from build123d import *

# Parameters (mm, degrees)
BOSS_EXTRUDE1_DEPTH = 3
SKETCH2_R           = 1.5
CUT_EXTRUDE3_DEPTH  = 3
CUT_EXTRUDE4_START  = -10
CUT_EXTRUDE4_DEPTH  = 10
BOSS_EXTRUDE2_START = -3
BOSS_EXTRUDE2_DEPTH = 3
SKETCH5_W           = 0.56
SKETCH5_H           = 32.898596714
CUT_EXTRUDE5_DEPTH  = 3
SKETCH6_W           = 0.2
SKETCH6_H           = 32.898596714
CUT_EXTRUDE6_DEPTH  = 3
SKETCH7_R           = 2
CUT_EXTRUDE8_DEPTH  = 3
BOSS_EXTRUDE3_START = -3
BOSS_EXTRUDE3_DEPTH = 3
CUT_EXTRUDE9_START  = -3
CUT_EXTRUDE9_DEPTH  = 3
BOSS_EXTRUDE5_START = -3
BOSS_EXTRUDE5_DEPTH = 3
SKETCH11_R          = 1.5
CUT_EXTRUDE10_DEPTH = 3
CUT_EXTRUDE11_DEPTH = 3
SKETCH13_W          = 7
SKETCH13_H          = 1.5
CUT_EXTRUDE12_DEPTH = 3
SKETCH14_R          = 2
SKETCH14_R_2        = 1.5
SKETCH14_W          = 7
SKETCH14_H          = 1.5
BOSS_EXTRUDE6_DEPTH = 3
CUT_EXTRUDE13_START = -2
CUT_EXTRUDE13_DEPTH = 2
SKETCH16_R          = 1.5
CUT_EXTRUDE14_DEPTH = 2


with BuildPart() as part:
    # Sketch1 → Boss-Extrude1 (new body)
    with BuildSketch(Plane.XY):
        with BuildLine():
            Line((-11, 25.5), (-22.790038711, 29.780264196))
            ThreePointArc((-22.790038711, 29.780264196), (0, -37.5), (22.790038711, 29.780264196))
            Line((22.790038711, 29.780264196), (11, 25.5))
            Line((11, 25.5), (-11, 25.5))
        make_face()
    extrude(amount=BOSS_EXTRUDE1_DEPTH)

    # Sketch2 → Cut-Extrude3 (cut)
    with BuildSketch(Plane.XY.offset(3)):
        with Locations((-25.400000001, 10.496905453)):
            Circle(SKETCH2_R)
        with Locations((-25.399981845, -10.493094547)):
            Circle(SKETCH2_R)
        with Locations(Location((25.399981845, -10.493094547, 0), (0, 0, 180))):
            Circle(SKETCH2_R)
        with Locations(Location((25.400000001, 10.496905453, 0), (0, 0, 180))):
            Circle(SKETCH2_R)
    extrude(amount=-CUT_EXTRUDE3_DEPTH, mode=Mode.SUBTRACT)

    # Sketch3 → Cut-Extrude4 (cut)
    with BuildSketch(Plane.XY.offset(3).offset(CUT_EXTRUDE4_START)):
        with BuildLine():
            Line((-30.76, 21.449298357), (-30.76, -21.449298357))
            ThreePointArc((-30.76, -21.449298357), (-37.5, 0), (-30.76, 21.449298357))
        make_face()
        with BuildLine():
            Line((30.76, 21.449298357), (30.76, -21.449298357))
            ThreePointArc((30.76, -21.449298357), (37.5, 0), (30.76, 21.449298357))
        make_face()
    extrude(amount=CUT_EXTRUDE4_DEPTH, mode=Mode.SUBTRACT)

    # Sketch4 → Boss-Extrude2 (add)
    with BuildSketch(Plane.XY.offset(3).offset(BOSS_EXTRUDE2_START)):
        with BuildLine():
            Line((-30.76, -21.449298357), (-30.76, -16.449298357))
            Line((-30.76, -16.449298357), (-33.699711921, -16.449298357))
            ThreePointArc((-33.699711921, -16.449298357), (-32.32667034, -19.006219634), (-30.76, -21.449298357))
        make_face()
        with BuildLine():
            Line((-33.699711921, 16.449298357), (-30.76, 16.449298357))
            Line((-30.76, 16.449298357), (-30.76, 21.449298357))
            ThreePointArc((-30.76, 21.449298357), (-32.32667034, 19.006219634), (-33.699711921, 16.449298357))
        make_face()
        with BuildLine():
            Line((30.76, 21.449298357), (30.76, 16.449298357))
            Line((30.76, 16.449298357), (33.699711921, 16.449298357))
            ThreePointArc((33.699711921, 16.449298357), (32.32667034, 19.006219634), (30.76, 21.449298357))
        make_face()
        with BuildLine():
            Line((30.76, -16.449298357), (30.76, -21.449298357))
            ThreePointArc((30.76, -21.449298357), (32.32667034, -19.006219634), (33.699711921, -16.449298357))
            Line((33.699711921, -16.449298357), (30.76, -16.449298357))
        make_face()
    extrude(amount=BOSS_EXTRUDE2_DEPTH)

    # Sketch5 → Cut-Extrude5 (cut)
    with BuildSketch(Plane.XY.offset(3)):
        with Locations((-30.48, 0)):
            Rectangle(SKETCH5_W, SKETCH5_H)
        with Locations((30.48, 0)):
            Rectangle(SKETCH5_W, SKETCH5_H)
    extrude(amount=-CUT_EXTRUDE5_DEPTH, mode=Mode.SUBTRACT)

    # Sketch6 → Cut-Extrude6 (cut)
    with BuildSketch(Plane.XY.offset(3)):
        with Locations((-30.1, 0)):
            Rectangle(SKETCH6_W, SKETCH6_H)
        with Locations((30.1, 0)):
            Rectangle(SKETCH6_W, SKETCH6_H)
    extrude(amount=-CUT_EXTRUDE6_DEPTH, mode=Mode.SUBTRACT)

    # Sketch7 → Cut-Extrude8 (cut)
    with BuildSketch(Plane.XY.offset(3)):
        with Locations((-19.15, -21.55)):
            Circle(SKETCH7_R)
        with Locations(Location((19.15, -21.55, 0), (0, 0, 180))):
            Circle(SKETCH7_R)
    extrude(amount=-CUT_EXTRUDE8_DEPTH, mode=Mode.SUBTRACT)

    # Sketch8 → Boss-Extrude3 (add)
    with BuildSketch(Plane.XY.offset(3).offset(BOSS_EXTRUDE3_START)):
        with BuildLine():
            Line((-33.699711921, 16.449298357), (-37.299711921, 16.449298357))
            ThreePointArc((-37.299711921, 16.449298357), (-32.744884003, 23.851322108), (-26.390038711, 29.780264196))
            Line((-26.390038711, 29.780264196), (-22.790038711, 29.780264196))
            ThreePointArc((-22.790038711, 29.780264196), (-29.020710607, 23.749702226), (-33.699711921, 16.449298357))
        make_face()
        with BuildLine():
            Line((33.699711921, 16.449298357), (37.299711921, 16.449298357))
            ThreePointArc((37.299711921, 16.449298357), (32.744884003, 23.851322108), (26.390038711, 29.780264196))
            Line((26.390038711, 29.780264196), (22.790038711, 29.780264196))
            ThreePointArc((22.790038711, 29.780264196), (29.020710607, 23.749702226), (33.699711921, 16.449298357))
        make_face()
    extrude(amount=BOSS_EXTRUDE3_DEPTH)

    # Sketch9 → Cut-Extrude9 (cut)
    with BuildSketch(Plane.XY.offset(3).offset(CUT_EXTRUDE9_START)):
        with BuildLine():
            Line((4.733920151, -37.2), (-4.733920151, -37.2))
            ThreePointArc((-4.733920151, -37.2), (0, -37.5), (4.733920151, -37.2))
        make_face()
    extrude(amount=CUT_EXTRUDE9_DEPTH, mode=Mode.SUBTRACT)

    # Sketch10 → Boss-Extrude5 (add)
    with BuildSketch(Plane.XY.offset(3).offset(BOSS_EXTRUDE5_START)):
        with BuildLine():
            ThreePointArc((-4.733920151, -37.2), (-21.838816892, -30.484685938), (-33.699711921, -16.449298357))
            Line((-33.699711921, -16.449298357), (-37.299711921, -16.449298357))
            ThreePointArc((-37.299711921, -16.449298357), (-23.43831182, -30.624902723), (-4.733920151, -37.2))
        make_face()
        with BuildLine():
            ThreePointArc((33.699711921, -16.449298357), (21.838816892, -30.484685938), (4.733920151, -37.2))
            ThreePointArc((4.733920151, -37.2), (23.43831182, -30.624902723), (37.299711921, -16.449298357))
            Line((37.299711921, -16.449298357), (33.699711921, -16.449298357))
        make_face()
        with BuildLine():
            Line((4.733920151, -37.2), (-4.733920151, -37.2))
            ThreePointArc((-4.733920151, -37.2), (0, -37.457659609), (4.733920151, -37.2))
        make_face()
    extrude(amount=BOSS_EXTRUDE5_DEPTH)

    # Sketch11 → Cut-Extrude10 (cut)
    with BuildSketch(Plane.XY.offset(3)):
        with Locations((-28.590038711, 23.780264196)):
            Circle(SKETCH11_R)
        with Locations(Location((28.590038711, 23.780264196, 0), (0, 0, 180))):
            Circle(SKETCH11_R)
    extrude(amount=-CUT_EXTRUDE10_DEPTH, mode=Mode.SUBTRACT)

    # Sketch12 → Cut-Extrude11 (cut)
    with BuildSketch(Plane.XY.offset(3)):
        Polygon((-22.005113558, -26.391105244), (-15.660959049, -29.349433076), (-16.294886442, -30.708894756), (-22.639040951, -27.750566924), align=None)
        Polygon((22.005113558, -26.391105244), (15.660959049, -29.349433076), (16.294886442, -30.708894756), (22.639040951, -27.750566924), align=None)
    extrude(amount=-CUT_EXTRUDE11_DEPTH, mode=Mode.SUBTRACT)

    # Sketch13 → Cut-Extrude12 (cut)
    with BuildSketch(Plane.XY.offset(3)):
        with Locations((-17.400000001, 9.496905453)):
            Rectangle(SKETCH13_W, SKETCH13_H)
        with Locations((17.400000001, 9.496905453)):
            Rectangle(SKETCH13_W, SKETCH13_H)
    extrude(amount=-CUT_EXTRUDE12_DEPTH, mode=Mode.SUBTRACT)

    # Sketch14 → Boss-Extrude6 (add)
    with BuildSketch(Plane.XY.offset(3)):
        with Locations((-19.15, -21.55)):
            Circle(SKETCH14_R)
        with Locations((19.15, -21.55)):
            Circle(SKETCH14_R)
        with Locations((-25.399981845, -10.493094547)):
            Circle(SKETCH14_R_2)
        with Locations((-25.400000001, 10.496905453)):
            Circle(SKETCH14_R_2)
        with Locations((25.400000001, 10.496905453)):
            Circle(SKETCH14_R_2)
        with Locations((25.399981845, -10.493094547)):
            Circle(SKETCH14_R_2)
        Polygon((-22.005113558, -26.391105244), (-22.639040951, -27.750566924), (-16.294886442, -30.708894756), (-15.660959049, -29.349433076), align=None)
        with Locations((-17.400000001, 9.496905453)):
            Rectangle(SKETCH14_W, SKETCH14_H)
        with Locations((17.400000001, 9.496905453)):
            Rectangle(SKETCH14_W, SKETCH14_H)
        Polygon((16.294886442, -30.708894756), (15.660959049, -29.349433076), (22.005113558, -26.391105244), (22.639040951, -27.750566924), align=None)
    extrude(amount=-BOSS_EXTRUDE6_DEPTH)

    # Sketch15 → Cut-Extrude13 (cut)
    with BuildSketch(Plane.XY.offset(3).offset(CUT_EXTRUDE13_START)):
        with BuildLine():
            Line((-37.299711921, 16.449298357), (-30, 16.449298357))
            Line((-30, 16.449298357), (-30, -16.449298357))
            Line((-30, -16.449298357), (-37.299711921, -16.449298357))
            ThreePointArc((-37.299711921, -16.449298357), (0, -37.457659609), (37.299711921, -16.449298357))
            Line((37.299711921, -16.449298357), (30, -16.449298357))
            Line((30, -16.449298357), (30, 16.449298357))
            Line((30, 16.449298357), (37.299711921, 16.449298357))
            ThreePointArc((37.299711921, 16.449298357), (32.744884003, 23.851322108), (26.390038711, 29.780264196))
            Line((26.390038711, 29.780264196), (22.790038711, 29.780264196))
            Line((22.790038711, 29.780264196), (11, 25.5))
            Line((11, 25.5), (-11, 25.5))
            Line((-11, 25.5), (-22.790038711, 29.780264196))
            Line((-22.790038711, 29.780264196), (-26.390038711, 29.780264196))
            ThreePointArc((-26.390038711, 29.780264196), (-32.744884003, 23.851322108), (-37.299711921, 16.449298357))
        make_face()
    extrude(amount=CUT_EXTRUDE13_DEPTH, mode=Mode.SUBTRACT)

    # Sketch16 → Cut-Extrude14 (cut)
    with BuildSketch(Plane.XY.offset(1)):
        with Locations((-31.299711921, -19.449298357)):
            Circle(SKETCH16_R)
        with Locations((31.299711921, -19.449298357)):
            Circle(SKETCH16_R)
    extrude(amount=-CUT_EXTRUDE14_DEPTH, mode=Mode.SUBTRACT)


solid = part.part
Geometry check sheet. Reference: the model listing, model coordinates, mm. A direction names the side the tool comes from. Round coordinates to 2 decimals unless told otherwise and drop trailing zeros. Loops run counter-clockwise (first coordinate to the right, second up) from the corner with the lowest first, then second, coordinate; pieces in that order, holes last. Notation, with made-up numbers: (3, 88) - (20, 88) arc R22 cw to (20, 119) - close; hole circle Ø1 at (42, 68). An arc over 180 degrees is marked (long way). Answer as CSV lines item,"result".
(1) Cross-section at D-D, the plane y = -8.5. Enter the section's corners in (x, z).
Output values:
outline,"(-30, 0) - (30, 0) - (30, 1) - (-30, 1) - close"
(2) Cross-section at B-B, the plane y = 26.5. Enter the section's corners in (x, z), and give its area (3 significant figures).
Output values:
outline,"(-30.32, 0) - (-13.75, 0) - (-13.75, 1) - (-30.32, 1) - close; (13.75, 0) - (30.32, 0) - (30.32, 1) - (13.75, 1) - close"
area,"33.1 mm²"
(3) Cross-section at A-A, the plane x = 28. Enter the section's corners in (y, z).
Output values:
outline,"(-27.28, 0) - (22.4, 0) - (22.4, 1) - (-27.28, 1) - close; (25.16, 0) - (28.56, 0) - (28.56, 1) - (25.16, 1) - close"
(4) Material ranges on line 1 along Y through (x, z) = (-31.5, 0.95); line 2 along X through (y, z) = (-16, 0.75); line 3 along X through (y, z) = (25, 0.2), recorded low to high.
Output values:
line 1,"y = -24.01 to -20.94, -17.96 to -16.45, 16.45 to 25.28"
line 2,"x = -30 to 30"
line 3,"x = -31.76 to -29.46, -27.72 to 27.72, 29.46 to 31.76"
(5) Set-up check for faces 1 (the face through (29.8, -19.4, 0.5)), 2 (the face through (16.98, 27.67, 0.49)): record each of +Z, -Z, +X, -X, +Y, -Y from which the full face is reachable in a straight line by a thin tool's end or side.
Output values:
face 1,"+Z, -Z"
face 2,"+Z, -Z, +Y"
(6) Cross-section at C-C, the plane z = 0.4. Enter the section's corners in (x, y), and give its area (3 significant figures).
Output values:
outline,"(-37.3, -16.45) arc R43.62 ccw to (37.3, -16.45) - (30, -16.45) - (30, 16.45) - (37.3, 16.45) arc R32.48 ccw to (26.39, 29.78) - (22.79, 29.78) - (11, 25.5) - (-11, 25.5) - (-22.79, 29.78) - (-26.39, 29.78) arc R32.48 ccw to (-37.3, 16.45) - (-30, 16.45) - (-30, -16.45) - close; hole circle Ø3 at (-31.3, -19.45); hole circle Ø3 at (-28.59, 23.78); hole circle Ø3 at (28.59, 23.78); hole circle Ø3 at (31.3, -19.45)"
area,"3,790 mm²"
(7) Release check for a two-part mould opening along Y. For faces 3 (the face through (29.7, 22.77, 0.51)), 4 (the face through (-1, -3, 0)), 5 (the face through (-32.82, 23.76, 0.49)) record: released by +Y, released by -Y, zero draft, split by the parting line, or undercut.
Output values:
face 3,"undercut"
face 4,"zero draft"
face 5,"released by +Y"
(8) Depth check by flat-ended pin: pin 1 Ø1.8 at (x, y) = (-31.3, -19.45) entering from -Z. Enter the tip coordinate at first touch or a pass-through.
Output values:
pin 1,"passes through"
